Could you check a few things on this model? Use its own coordinates, in mm. A direction names the side the tool comes from. Coordinates: 2 decimals unless noted, no trailing zeros. Loops run counter-clockwise (first coordinate to the right, second up) from the corner with the lowest first, then second, coordinate; pieces in that order, holes last.
from build123d import *

# Parameters (mm, degrees)
SKETCH2_W               = 60
SKETCH2_H               = 60
BOSS_EXTRUDE1_DEPTH     = 20
SKETCH9_R               = 8.5
SKETCH10_RX             = 8.5
SKETCH10_RY             = 6.01040764
SKETCH12_R              = 3
CUT_EXTRUDE1_DEPTH      = 61
SKETCH13_R              = 3
CUT_EXTRUDE2_DEPTH      = 21
SKETCH15_W              = 5
SKETCH15_H              = 15.5
BOSS_EXTRUDE2_DEPTH     = 20
FILLET1_R               = 10
SKETCH17_W              = 28.111929505
SKETCH17_H              = 1
CUT_EXTRUDE3_DEPTH      = 23
CUT_EXTRUDE3_DEPTH_BACK = 3


with BuildPart() as part:
    # Sketch2 → Boss-Extrude1 (new body)
    with BuildSketch(Plane(origin=(0, 0, 0), x_dir=(1, 0, 0), z_dir=(0, 1, 0))):
        Rectangle(SKETCH2_W, SKETCH2_H)
    extrude(amount=BOSS_EXTRUDE1_DEPTH)

    # Sketch9 → Loft1 section 0
    with BuildSketch(Plane(origin=(15, 15, 0), x_dir=(0, 0, -1), z_dir=(0.707106781, 0.707106781, 0))):
        with Locations((0, 21.213203436)):
            Circle(SKETCH9_R)
    # Sketch10 → Loft1 section 1
    with BuildSketch(Plane(origin=(0, 20, 0), x_dir=(1, 0, 0), z_dir=(0, 1, 0))):
        with Locations(Location((0, 0), (0, 0, 90))):
            Ellipse(SKETCH10_RX, SKETCH10_RY)
    loft()

    # Sketch12 → Cut-Extrude1 (cut, through all)
    with BuildSketch(Plane(origin=(30, 0, 0), x_dir=(0, 0, -1), z_dir=(1, 0, 0))):
        with Locations((0, 30)):
            Circle(SKETCH12_R)
    extrude(amount=-CUT_EXTRUDE1_DEPTH, mode=Mode.SUBTRACT)

    # Sketch13 → Cut-Extrude2 (cut, through all)
    with BuildSketch(Plane(origin=(0, 20, 0), x_dir=(1, 0, 0), z_dir=(0, 1, 0))):
        Circle(SKETCH13_R)
    extrude(amount=-CUT_EXTRUDE2_DEPTH, mode=Mode.SUBTRACT)

    # Sketch15 → Boss-Extrude2 (add)
    with BuildSketch(Plane(origin=(0, 20, 0), x_dir=(1, 0, 0), z_dir=(0, 1, 0))):
        with Locations((-27.5, 0)):
            Rectangle(SKETCH15_W, SKETCH15_H)
    extrude(amount=BOSS_EXTRUDE2_DEPTH)

    # Fillet1
    fillet1_edges = [part.edges().sort_by_distance(p)[0] for p in [
        (-27.5, 20, 7.75),
        (-27.5, 20, -7.75),
    ]]
    fillet(fillet1_edges, radius=FILLET1_R)

    # Sketch17 → Cut-Extrude3 (cut, two sides)
    with BuildSketch(Plane(origin=(-8.98959236, 8.98959236, 0), x_dir=(0, 0, 1), z_dir=(-0.707106781, 0.707106781, 0))) as cut_extrude3_sk:
        with Locations((0.173110945, 20.713203436)):
            Rectangle(SKETCH17_W, SKETCH17_H)
    extrude(amount=CUT_EXTRUDE3_DEPTH, mode=Mode.SUBTRACT)
    extrude(cut_extrude3_sk.sketch, amount=-CUT_EXTRUDE3_DEPTH_BACK, mode=Mode.SUBTRACT)


solid = part.part
(1) Imagine slicing it at B-B, the plane z = -16. Write out the boundary of the cut face in (x, y), and give its area (3 significant figures).
Answers:
outline: (-30, 0) - (30, 0) - (30, 20) - (-25, 20) - (-25, 20.15) - (-30, 20.15) - close
area: 1,200 mm2
(2) Imagine slicing it at D-D, the plane x = 16. Write out the boundary of the cut face in (y, z).
Answers:
outline: (0, -30) - (20, -30) - (20, 30) - (0, 30) - close
(3) Imagine slicing it at A-A, the plane x = -26. Write out the boundary of the cut face in (y, z), and give its area (3 significant figures).
Answers:
outline: (0, -30) - (20, -30) - (20, -17.75) arc R10 cw to (30, -7.75) - (40, -7.75) - (40, 7.75) - (30, 7.75) arc R10 cw to (20, 17.75) - (20, 30) - (0, 30) - close
area: 1,550 mm2
(4) Which directions (+Z, -Z, +X, -X, +Y, -Y) give clear straight access to the entire face, cutting with the end or side of a thin tool? Please do faces 4 (the face through (-27.46, 22.85, -10.76)), 5 (the face through (-25, 30, 0)), 6 (the face through (-27.46, 22.85, 10.76)), 7 (the face through (-3, 10, 0)), 8 (the face through (-2.97, 27.07, 0.65)).
Answers:
face 4: -Z, -X, +Y
face 5: +Z, -Z, +Y
face 6: +Z, -X, +Y
face 7: -Y
face 8: +X
(5) I need wall thicknesses on probe 1 along X at (y, z) = (15, 0); probe 2 along X at (y, z) = (31, -2). Which ranges of each line are inside material? Lowest first, please.
Answers:
probe 1: x = -30 to -3, 3 to 30
probe 2: x = -30 to -25
(6) For pin 1 (1.5 mm diameter, centred on x = 22, z = 16.5, fed in from -Y); pin 2 (4 mm diameter, centred on x = -27.5, y = 36.5, fed in from +Z); pin 3 (1 mm diameter, centred on x = -2.5, z = -20.5, fed in from +Y); pin 4 (1 mm diameter, centred on y = 31, z = 9, fed in from +X), each with a flat end and sliding along its axis, tell me the tip position at first contact or that it passes through.
Answers:
pin 1: stops at y = 0
pin 2: stops at z = 7.75
pin 3: stops at y = 20
pin 4: passes through
(7) Imagine slicing it at C-C, the plane z = 26.5. Write out the boundary of the cut face in (x, y).
Answers:
outline: (-30, 0) - (30, 0) - (30, 20) - (-30, 20) - close
(8) We'd pull the mould along X, two halves only. Please class faces 1 (the face through (30, 10, 0)), 2 (the face through (-7, 0, 0)), 3 (the face through (0, 20, 0)): +X half, -X half, draft (parallel to the pull), parting line (faces both ways), or undercut.
Answers:
face 1: +X half
face 2: draft
face 3: undercut
